```python
from build123d import *

# Parameters (mm, degrees)
SKETCH_1_W          = 80
SKETCH_1_H          = 60.5
EXTRUDE_1_DEPTH     = 5
SKETCH_3_R          = 19.05
CUT_EXTRUDE_1_DEPTH = 52.137681801
HOLE_WIZARD_M4_1_D  = 4.5
HOLE_WIZARD_M5_1_D  = 5.3


with BuildPart() as part:
    # 草圖1 → 填料-伸長1 (new, symmetric)
    with BuildSketch(Plane.XY):
        Rectangle(SKETCH_1_W, SKETCH_1_H)
    extrude(amount=EXTRUDE_1_DEPTH, both=True)

    # 草圖3 → 除料-伸長1 (cut, through all)
    with BuildSketch(Plane.XY.offset(5)):
        Circle(SKETCH_3_R)
    extrude(amount=-CUT_EXTRUDE_1_DEPTH, mode=Mode.SUBTRACT)

    # M4 餘隙孔1 (through all)
    with Locations(Plane(origin=(0, 0, -5), x_dir=(-1, 0, 0), z_dir=(0, 0, -1))):
        with Locations((23.57, 23.57), (-23.57, -23.57), (-23.57, 23.57), (23.57, -23.57)):
            Hole(HOLE_WIZARD_M4_1_D / 2)

    # M5 餘隙孔1 (through all)
    with Locations(Plane(origin=(0, 30.25, 0), x_dir=(1, 0, 0), z_dir=(0, 1, 0))):
        with Locations((-35, 0), (35, 0)):
            Hole(HOLE_WIZARD_M5_1_D / 2)


solid = part.part
```
Here's how the part is built. I have some questions about the finished solid (model axes, mm). Coordinates: 2 decimals unless noted, no trailing zeros. Loops run counter-clockwise (first coordinate to the right, second up) from the corner with the lowest first, then second, coordinate; pieces in that order, holes last. Notation, with made-up numbers: (-14, 58) - (16, 58) arc R18 cw to (16, 78) - close; hole circle Ø3 at (-35, 42.25). An arc over 180 degrees is marked (long way). Answer as CSV lines item,"result".
Q1. If we section it at A-A, the plane y = -23.57: Write out the boundary of the cut face in (x, z).
Response:
outline,"(-40, -5) - (-25.82, -5) - (-25.82, 5) - (-40, 5) - close; (-21.32, -5) - (21.32, -5) - (21.32, 5) - (-21.32, 5) - close; (25.82, -5) - (40, -5) - (40, 5) - (25.82, 5) - close; hole circle Ø5.3 at (-35, 0); hole circle Ø5.3 at (35, 0)"
Q2. For pin 1 (6 mm diameter, centred on x = 23.57, y = -23.57, fed in from +Z), with a flat end and sliding along its axis, tell me the tip position at first contact or that it passes through.
Response:
pin 1,"z = 5"
Q3. We'd pull the mould along X, two halves only. Please class faces 1 (the face through (-40, 0, 0)), 2 (the face through (21.322, -23.471, 0.07)), 3 (the face through (-22.36, 25.467, 0.07)), 4 (the face through (40, 0, 0)): pulls with the +X half, pulls with the -X half, needs draft (parallel to the pull), parting line crosses it, or undercut.
Response:
face 1,"pulls with the -X half"
face 2,"undercut"
face 3,"undercut"
face 4,"pulls with the +X half"
Q4. If I drill on L1, parallel to Y at x = 23.57, z = 1.75; L2, parallel to Y at x = 0, z = -2; L3, parallel to Y at x = 23, z = 2.5, over which ranges is the centre line in solid material (lowest first)? Write a range as [from, to].
Response:
L1,"[-30.25, -25.82], [-21.32, 21.32], [25.82, 30.25]"
L2,"[-30.25, -19.05], [19.05, 30.25]"
L3,"[-30.25, -25.75], [-21.39, 21.39], [25.75, 30.25]"
Q5. If we section it at B-B, the plane x = -35: Write out the boundary of the cut face in (y, z).
Response:
outline,"(-30.25, -5) - (30.25, -5) - (30.25, -2.65) - (-30.25, -2.65) - close; (-30.25, 2.65) - (30.25, 2.65) - (30.25, 5) - (-30.25, 5) - close"
Q6. If we section it at C-C, the plane y = -10.5: Write out the boundary of the cut face in (x, z), and give its area (3 significant figures).
Response:
outline,"(-40, -5) - (-15.9, -5) - (-15.9, 5) - (-40, 5) - close; (15.9, -5) - (40, -5) - (40, 5) - (15.9, 5) - close; hole circle Ø5.3 at (-35, 0); hole circle Ø5.3 at (35, 0)"
area,"438 mm2"
Q7. If we section it at D-D, the plane z = 3.5: Write out the boundary of the cut face in (x, y).
Response:
outline,"(-40, -30.25) - (40, -30.25) - (40, 30.25) - (-40, 30.25) - close; hole circle Ø4.5 at (-23.57, -23.57); hole circle Ø4.5 at (-23.57, 23.57); hole circle Ø38.1 at (0, 0); hole circle Ø4.5 at (23.57, -23.57); hole circle Ø4.5 at (23.57, 23.57)"
